The listing builds one solid part. Answer for the finished solid, in the listing's coordinates (mm). A direction names the side the tool comes from. Coordinates: 2 decimals unless noted, no trailing zeros. Loops run counter-clockwise (first coordinate to the right, second up) from the corner with the lowest first, then second, coordinate; pieces in that order, holes last. Notation, with made-up numbers: M 2,84 L 50,84 A32 cw 50,110 Z; hole C -18.75,70 d5. An arc over 180 degrees is marked long. Answer as a JSON object with one key per item and string values. Group by question number.
1. Given pin 1 (11 mm diameter, centred on x = 44.5, z = 73.5, fed in from +Y); pin 2 (5 mm diameter, centred on x = -75, y = 15, fed in from +Z); pin 3 (2 mm diameter, centred on x = -72.5, y = 9.5, fed in from +Z), each flat-ended and moving along its own axis, determine where each tip first touches the part or whether it passes through.
2. A cutting plane is placed at D-D on z = 45. Give the vertices of the cut face in (x, y).
3. A cutting plane is placed at B-B on x = 36. Give the vertices of the cut face in (y, z), and give its area (3 significant figures).
4. For faces 4 (the face through (-74, -35, 27)), 5 (the face through (41, 14, 26)), 6 (the face through (-15, -22, 2)), determine the directions among +Z, -Z, +X, -X, +Y, -Y from which every point of the face is accessible in a straight line to the end or side of a thin tool.
5. A cutting plane is placed at C-C on z = 99.5. Give the vertices of the cut face in (x, y).
6. Determine the mould class of faces 1 (the face through (46, 16, 67)), 2 (the face through (51, -39.2, 44.4)), 3 (the face through (-69, 14, 26)) for opening direction X: released by +X, released by -X, zero draft, split by the parting line, or undercut.
7. A cutting plane is placed at A-A on z = 14. Give the vertices of the cut face in (x, y), and give its area (3 significant figures).
8. Straight lines are drawn through the part: L1, parallel to X at y = -42, z = 78; L2, parallel to Z at x = 44.5, y = -29. For each, find the intervals that lie inside material, in ascending order.
from build123d import *

# Parameters (mm, degrees)
SKETCH_W     = 110
SKETCH_H     = 18
PAD_DEPTH    = 5
SKETCH001_W  = 10
SKETCH001_H  = 13
PAD001_DEPTH = 22
SKETCH002_W  = 10
SKETCH002_H  = 6
PAD002_DEPTH = 40
SKETCH003_W  = 10
SKETCH003_H  = 6
PAD003_DEPTH = 100


with BuildPart() as part:
    # Sketch → Pad (new body)
    with BuildSketch(Plane(origin=(-14, -13, 0), x_dir=(1, 0, 0), z_dir=(0, 0, 1))):
        Polygon((-55, 19), (55, 19), (55, 32), (65, 32), (65, -32), (55, -32), (55, -19), (-55, -19), (-55, -32), (-65, -32), (-65, 32), (-55, 32), align=None)
        Rectangle(SKETCH_W, SKETCH_H, mode=Mode.SUBTRACT)
    extrude(amount=PAD_DEPTH)

    # Sketch001 → Pad001 (new body)
    with BuildSketch(Plane(origin=(-14, -13, 5), x_dir=(1, 0, 0), z_dir=(0, 0, 1))):
        with Locations((-60, 25.5)):
            Rectangle(SKETCH001_W, SKETCH001_H)
        with Locations((-60, -25.5)):
            Rectangle(SKETCH001_W, SKETCH001_H)
        with Locations((60, 25.5)):
            Rectangle(SKETCH001_W, SKETCH001_H)
        with Locations((60, -25.5)):
            Rectangle(SKETCH001_W, SKETCH001_H)
    extrude(amount=PAD001_DEPTH)

    # Sketch002 → Pad002 (new body)
    with BuildSketch(Plane(origin=(-14, -13, 27), x_dir=(1, 0, 0), z_dir=(0, 0, 1))):
        with Locations((-60, 29)):
            Rectangle(SKETCH002_W, SKETCH002_H)
    pad002 = extrude(amount=PAD002_DEPTH)

    # Mirrored: Pad002 across Sketch002 V_Axis
    add(pad002.mirror(Plane(origin=(-14, -13, 27), x_dir=(0, 0, 1), z_dir=(1, 0, 0))))

    # Sketch003 → Pad003 (new body)
    with BuildSketch(Plane(origin=(-14, -13, 27), x_dir=(1, 0, 0), z_dir=(0, 0, 1))):
        with Locations((-60, -29)):
            Rectangle(SKETCH003_W, SKETCH003_H)
    pad003 = extrude(amount=PAD003_DEPTH)

    # Mirrored001: Pad003 across Sketch003 V_Axis
    add(pad003.mirror(Plane(origin=(-14, -13, 27), x_dir=(0, 0, 1), z_dir=(1, 0, 0))))


solid = part.part
From the geometry:
{
 "1": {"pin 1": "stops at y = -39", "pin 2": "stops at z = 67", "pin 3": "stops at z = 27"},
 "2": {"outline": "M -79,-45 L -69,-45 L -69,-39 L -79,-39 Z; M -79,13 L -69,13 L -69,19 L -79,19 Z; M 41,-45 L 51,-45 L 51,-39 L 41,-39 Z; M 41,13 L 51,13 L 51,19 L 41,19 Z"},
 "3": {"outline": "M -32,0 L -22,0 L -22,5 L -32,5 Z; M -4,0 L 6,0 L 6,5 L -4,5 Z", "area": "100 mm²"},
 "4": {"face 4": "+Z, +X, -X", "face 5": "+Z, -Z, +Y", "face 6": "+Z, -Z"},
 "5": {"outline": "M -79,-45 L -69,-45 L -69,-39 L -79,-39 Z; M 41,-45 L 51,-45 L 51,-39 L 41,-39 Z"},
 "6": {"face 1": "zero draft", "face 2": "released by +X", "face 3": "undercut"},
 "7": {"outline": "M -79,-45 L -69,-45 L -69,-32 L -79,-32 Z; M -79,6 L -69,6 L -69,19 L -79,19 Z; M 41,-45 L 51,-45 L 51,-32 L 41,-32 Z; M 41,6 L 51,6 L 51,19 L 41,19 Z", "area": "520 mm²"},
 "8": {"L1": "x = -79 to -69, 41 to 51", "L2": "z = 0 to 5"}
}
